from build123d import *

# Parameters (mm, degrees)
SKETCH1_R                = 28
BOSS_EXTRUDE1_DEPTH      = 9
SKETCH2_R                = 11
CUT_EXTRUDE1_DEPTH       = 3
SKETCH3_R                = 9
CUT_EXTRUDE2_DEPTH       = 16
SKETCH4_R                = 11
CUT_EXTRUDE3_DEPTH       = 6.5
SKETCH_1_R               = 2.5
CUT_EXTRUDE_1_DEPTH      = 19
PATTERN_CIRCULAR_1_COUNT = 6


with BuildPart() as part:
    # Sketch1 → Boss-Extrude1 (new body, symmetric)
    with BuildSketch(Plane.XY):
        Circle(SKETCH1_R)
    extrude(amount=BOSS_EXTRUDE1_DEPTH, both=True)

    # Sketch2 → Cut-Extrude1 (cut)
    with BuildSketch(Plane.XY.offset(9)):
        Circle(SKETCH2_R)
    extrude(amount=-CUT_EXTRUDE1_DEPTH, mode=Mode.SUBTRACT)

    # Sketch3 → Cut-Extrude2 (cut, through all)
    with BuildSketch(Plane.XY.offset(6)):
        Circle(SKETCH3_R)
    extrude(amount=-CUT_EXTRUDE2_DEPTH, mode=Mode.SUBTRACT)

    # Sketch4 → Cut-Extrude3 (cut)
    with BuildSketch(Plane(origin=(0, 0, -9), x_dir=(-1, 0, 0), z_dir=(0, 0, -1))):
        Circle(SKETCH4_R)
    extrude(amount=-CUT_EXTRUDE3_DEPTH, mode=Mode.SUBTRACT)

    # 草圖1 → 除料-伸長1 (cut, through all)
    with BuildSketch(Plane.XY.offset(9)):
        with Locations((0, 23.75)):
            Circle(SKETCH_1_R)
    cut_extrude_1 = extrude(amount=-CUT_EXTRUDE_1_DEPTH, mode=Mode.SUBTRACT)

    # 環狀複製排列1: 除料-伸長1 ×6 about axis
    pattern_circular_1_axis = Axis((0, 0, 0), (0, 0, 1))
    for i in range(1, PATTERN_CIRCULAR_1_COUNT):
        add(cut_extrude_1.rotate(pattern_circular_1_axis, i * 360 / PATTERN_CIRCULAR_1_COUNT), mode=Mode.SUBTRACT)


solid = part.part
Could you check a few things on this model? Use its own coordinates, in mm. A direction names the side the tool comes from. Round coordinates to 2 decimals unless told otherwise and drop trailing zeros. Loops run counter-clockwise (first coordinate to the right, second up) from the corner with the lowest first, then second, coordinate; pieces in that order, holes last. Notation, with made-up numbers: (-37.5, 88) - (-20.5, 88) arc R22 ccw to (-20.5, 124) - close; hole circle Ø3 at (-11, 65). An arc over 180 degrees is marked (long way). Write item = value, one per line.
1) I need wall thicknesses on line 1 along Y through (x, z) = (0, 8); line 2 along Y through (x, z) = (0, -0.5); line 3 along Y through (x, z) = (20, -1.5). Which ranges of each line are inside material? Lowest first, please. Write a range as from..to.
Computed:
line_1 = -28..-26.25, -21.25..-11, 11..21.25, 26.25..28
line_2 = -28..-26.25, -21.25..-9, 9..21.25, 26.25..28
line_3 = -19.6..-14.31, -9.44..9.44, 14.31..19.6
2) On a 3-axis mill with a long thin cutter (end or side, diameter ignored), from which of +Z, -Z, +X, -X, +Y, -Y can I reach the whole of each face in a straight line? I mean faces 5 (the cylindrical face through (-2.38, -10.74, 7.52)), 6 (the cylindrical face through (2.38, -10.74, -5.8)), 7 (the flat face through (12, 0, -9)). Say none if no direction works.
Computed:
face_5 = +Z
face_6 = -Z
face_7 = -Z, +X, -X, +Y, -Y
3) If we mould it in two halves opening along X, with no side actions, what happens to faces 1 (the cylindrical face through (0.33, -26.23, 0.13)), 2 (the cylindrical face through (-1.172, 8.923, 1.81)), 3 (the cylindrical face through (25.865, -10.724, 0.126)), 4 (the flat face through (12, 0, 9))? For each: pulls with the +X half, pulls with the -X half, needs draft (parallel to the pull), parting line crosses it, or undercut.
Computed:
face_1 = undercut
face_2 = undercut
face_3 = parting line crosses it
face_4 = needs draft
4) Imagine slicing it at D-D (y = 23.75). Please give me the cut outline in (x, z).
Computed:
outline = (-14.83, -9) - (-2.5, -9) - (-2.5, 9) - (-14.83, 9) - close; (2.5, -9) - (14.83, -9) - (14.83, 9) - (2.5, 9) - close
5) Imagine slicing it at B-B (x = 4). Please give me the cut outline in (y, z).
Computed:
outline = (-27.71, -9) - (-10.25, -9) - (-10.25, -2.5) - (-8.06, -2.5) - (-8.06, 6) - (-10.25, 6) - (-10.25, 9) - (-27.71, 9) - close; (8.06, -2.5) - (10.25, -2.5) - (10.25, -9) - (27.71, -9) - (27.71, 9) - (10.25, 9) - (10.25, 6) - (8.06, 6) - close
6) I'm going to push flat-ended pins straight in: P1, Ø16, axis at x = 0, y = 0, coming from the +Z side; P2, Ø4, axis at x = -7.5, z = -6.5, coming from the +Y side; P3, Ø1.5, axis at x = -18.5, z = -3, coming from the -Y side; P4, Ø1, axis at x = -22, z = 3, coming from the -Y side. Where does each tip first touch, or does it pass through?
Computed:
P1 = through
P2 = 27.45
P3 = -21.65
P4 = -17.94
7) Imagine slicing it at A-A (y = 0). Please give me the cut outline in (x, z).
Computed:
outline = (-28, -9) - (-11, -9) - (-11, -2.5) - (-9, -2.5) - (-9, 6) - (-11, 6) - (-11, 9) - (-28, 9) - close; (9, -2.5) - (11, -2.5) - (11, -9) - (28, -9) - (28, 9) - (11, 9) - (11, 6) - (9, 6) - close
8) Imagine slicing it at C-C (z = 0). Please give me the cut outline in (x, y) (3 decimals).
Computed:
outline = circle Ø56 at (0, 0); hole circle Ø5 at (-20.568, -11.875); hole circle Ø5 at (-20.568, 11.875); hole circle Ø18 at (0, 0); hole circle Ø5 at (0, -23.75); hole circle Ø5 at (0, 23.75); hole circle Ø5 at (20.568, -11.875); hole circle Ø5 at (20.568, 11.875)
